```python
from build123d import *

# Parameters (mm, degrees)
SKETCH1_W                 = 44
SKETCH1_H                 = 29
BOSS_EXTRUDE1_DEPTH       = 57.6
SKETCH2_R                 = 14.5
BOSS_EXTRUDE2_DEPTH       = 32
M3X0_5_TAPPED_HOLE1_D     = 2.5
M3X0_5_TAPPED_HOLE1_DEPTH = 3
M3X0_5_TAPPED_HOLE1_TIP   = 0.751075774


with BuildPart() as part:
    # Sketch1 → Boss-Extrude1 (new body)
    with BuildSketch(Plane.XY):
        Rectangle(SKETCH1_W, SKETCH1_H)
    extrude(amount=BOSS_EXTRUDE1_DEPTH)

    # Sketch2 → Boss-Extrude2 (add)
    with BuildSketch(Plane.XY):
        Circle(SKETCH2_R)
    extrude(amount=-BOSS_EXTRUDE2_DEPTH)

    # M3x0.5 Tapped Hole1
    with Locations(Plane(origin=(0, 14.5, 0), x_dir=(1, 0, 0), z_dir=(0, 1, 0))):
        with Locations((-13, -5), (13, -5)):
            Hole(M3X0_5_TAPPED_HOLE1_D / 2, depth=M3X0_5_TAPPED_HOLE1_DEPTH)
            with Locations((0, 0, -(M3X0_5_TAPPED_HOLE1_DEPTH + M3X0_5_TAPPED_HOLE1_TIP / 2))):  # 118° drill point
                Cone(0, M3X0_5_TAPPED_HOLE1_D / 2, M3X0_5_TAPPED_HOLE1_TIP, mode=Mode.SUBTRACT)


solid = part.part
```
Read the model definition and answer for the solid it produces. Units are mm, in the model's axes. A direction names the side the tool comes from. Give positions to 0.01 mm unless a question says otherwise; leave off trailing zeros. Write each loop counter-clockwise with the first axis right and the second up, starting at its lowest first coordinate (ties: lowest second). Pieces come first, ordered by that corner, then holes. Notation, with made-up numbers: M -18,-19 L 27,-19 A11 cw 27,-15 Z; hole C 33,40.5 d6. An arc over 180 degrees is marked long. Put each result on its own line as item: value. Start each with the question number.
1. The part is cut by section A-A, the plane y = 0. Give the vertices of the cut face in (x, z), and give its area (3 significant figures).
2. The part is cut by section B-B, the plane x = -18.5. Give the vertices of the cut face in (y, z), and give its area (3 significant figures).
3. Which of the six approach directions +Z, -Z, +X, -X, +Y, -Y give full straight-line access (tool end or side, diameter ignored) to faces 4 (the flat face through (-16, 0, 0)), 5 (the cylindrical face through (-12.73, 12.98, 6.22)), 6 (the cylindrical face through (6.691, -12.864, -15.776))?
4. Consider line 1 along X through (y, z) = (13.7, 5); line 2 along Z through (x, y) = (-13, 13); line 3 along Y through (x, z) = (-8.5, -14.5). Determine where each line is inside the solid, lowest interval first.
5. Each of these flat-tipped pins is pushed along its axis until it touches: pin 1 Ø6 at (x, z) = (3.5, -8.5) entering from -Y; pin 2 Ø8 at (y, z) = (-4.5, -13) entering from +X; pin 3 Ø1 at (x, z) = (-4.5, -18.5) entering from +Y. Where does it stop, or does it pass through?
6. The part is cut by section C-C, the plane y = 4.5. Give the vertices of the cut face in (x, z), and give its area (3 significant figures).
7. For a pull along Z with two mould halves and no side action, classify faces 1 (the flat face through (16, 0, 0)), 2 (the flat face through (22, 0, 28)), 3 (the cylindrical face through (13.99, 12.98, 5.76)) as released by +Z, released by -Z, zero draft, split by the parting line, or undercut.
Final values:
1. outline: M -22,0 L -14.5,0 L -14.5,-32 L 14.5,-32 L 14.5,0 L 22,0 L 22,57.6 L -22,57.6 Z
1. area: 3,460 mm²
2. outline: M -14.5,0 L 14.5,0 L 14.5,57.6 L -14.5,57.6 Z
2. area: 1,670 mm²
3. face 4: -Z, -X
3. face 5: +Y
3. face 6: -Z
4. line 1: x = -22 to -14.25, -11.75 to 11.75, 14.25 to 22
4. line 2: z = 0 to 3.75, 6.25 to 57.6
4. line 3: y = -11.75 to 11.75
5. pin 1: stops at y = -14.49
5. pin 2: stops at x = 14.49
5. pin 3: stops at y = 13.94
6. outline: M -22,0 L -13.78,0 L -13.78,-32 L 13.78,-32 L 13.78,0 L 22,0 L 22,57.6 L -22,57.6 Z
6. area: 3,420 mm²
7. face 1: released by -Z
7. face 2: zero draft
7. face 3: undercut
